For this review, use the dimensioned drawing (mm, ordinates from the lowest corner) and the shaded views. A direction names the side the tool comes from. Coordinates: 2 decimals unless noted, no trailing zeros. Loops run counter-clockwise (first coordinate to the right, second up) from the corner with the lowest first, then second, coordinate; pieces in that order, holes last. Notation, with made-up numbers: (41, -16.75) -> (51, -16.75) arc R23 cw to (51, -4.75) -> close; hole circle Ø6 at (-30.5, 24). An arc over 180 degrees is marked (long way). Use one line per item in the form item = value. Start each with the question number.
1. Consider section C-C (y = 22). State the section outline as (x, z) points (3 decimals).
2. Wall thickness on line 1 (X direction, y = 30, z = 39); line 2 (Z direction, x = 12.75, y = 42); line 3 (Z direction, x = 14.5, y = 44.5): over which ranges is each line inside the solid? List them lowest first. Write a range as from..to.
3. For pin 1 (12 mm diameter, centred on x = 9.5, y = 6.5, fed in from +Z); pin 2 (22 mm diameter, centred on y = 6, z = 32.5, fed in from +X); pin 3 (1 mm diameter, centred on x = 1, y = 4.5, fed in from +Z); pin 4 (5.5 mm diameter, centred on x = 11.75, z = 12, fed in from -Y), all flat-tipped, find the tip position at first contact; note any pin that passes through.
4. Machinability: for the marked faces 1 and 2, which of the approach directions +Z, -Z, +X, -X, +Y, -Y give a long, thin tool a straight path to every point of the face, cutting with its end or side? Answer none if there is none.
5. Consider section D-D (z = 32.5). State the section outline as (x, y) points.
6. The part is to be moulded in two halves that separate along X. For the marked faces 3, 4 and 5, say which applies: released by +X, released by -X, zero draft, split by the parting line, or undercut.
7. Consider section A-A (x = 11.75). State the section outline as (y, z) points (3 decimals).
8. Consider section B-B (z = 39). State the section outline as (x, y) points.
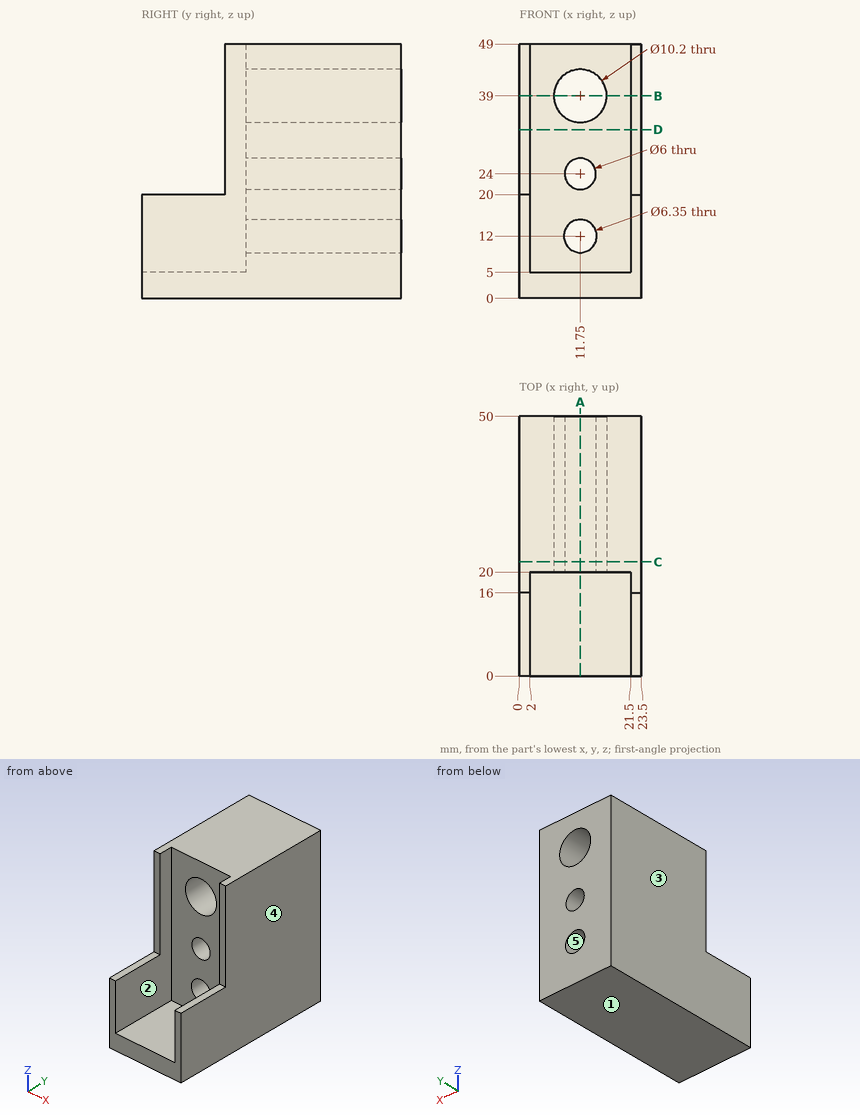
Geometry check:
q1.outline = (0, 0) -> (23.5, 0) -> (23.5, 49) -> (0, 49) -> close; hole circle Ø10.2 at (11.75, 39); hole circle Ø6.35 at (11.75, 12); hole circle Ø6 at (11.75, 24)
q2.line_1 = 0..6.65, 16.85..23.5
q2.line_2 = 0..8.99, 15.01..21.17, 26.83..34, 44..49
q2.line_3 = 0..10.41, 13.59..22.8, 25.2..34.7, 43.3..49
q3.pin_1 = 5
q3.pin_2 = 23.5
q3.pin_3 = 20
q3.pin_4 = through
q4.face_1 = -Z, +X, -X, +Y, -Y
q4.face_2 = +Z, -Y
q5.outline = (0, 16) -> (2, 16) -> (2, 20) -> (21.5, 20) -> (21.5, 16) -> (23.5, 16) -> (23.5, 50) -> (0, 50) -> close
q6.face_3 = released by -X
q6.face_4 = released by +X
q6.face_5 = undercut
q7.outline = (0, 0) -> (50, 0) -> (50, 8.825) -> (20, 8.825) -> (20, 5) -> (0, 5) -> close; (20, 15.175) -> (50, 15.175) -> (50, 21) -> (20, 21) -> close; (20, 27) -> (50, 27) -> (50, 33.9) -> (20, 33.9) -> close; (20, 44.1) -> (50, 44.1) -> (50, 49) -> (20, 49) -> close
q8.outline = (0, 16) -> (2, 16) -> (2, 20) -> (6.65, 20) -> (6.65, 50) -> (0, 50) -> close; (16.85, 20) -> (21.5, 20) -> (21.5, 16) -> (23.5, 16) -> (23.5, 50) -> (16.85, 50) -> close
